Model file for the job. Use its own axes, mm. A direction names the side the tool comes from. Round coordinates to 2 decimals unless told otherwise and drop trailing zeros. Loops run counter-clockwise (first coordinate to the right, second up) from the corner with the lowest first, then second, coordinate; pieces in that order, holes last. Notation, with made-up numbers: (-0.75, 59) - (57.25, 59) arc R27 cw to (57.25, 86) - close; hole circle Ø1 at (21, 3). An arc over 180 degrees is marked (long way). Answer as a JSON object with one key per item and string values.
from build123d import *

# Parameters (mm, degrees)
F1_DEPTH = 127
F3_DEPTH = 177.8
F4_R     = 33.3375
F4_R_2   = 31.75
F5_DEPTH = 19.05
F6_T     = 7.62


# Not quite as in the source:
# - a shell that OpenCascade refuses in one call is made with other operations: the cavity is built on its own and cut out


with BuildPart() as f1:
    # F0 (on Right) → F1 (new body, symmetric)
    with BuildSketch(Plane.YZ):
        with BuildLine():
            Line((0, 76.4100525974), (0, 0))
            Line((0, 0), (671.8020987012, 0))
            ThreePointArc((671.8020987012, 0), (693.9200398628, 12.9117383606), (693.5512826501, 38.5199465532))
            Line((693.5512826501, 38.5199465532), (616.9399846733, 165.5199465532))
            ThreePointArc((616.9399846733, 165.5199465532), (607.6790623638, 174.5179411616), (595.1908007244, 177.8))
            Line((595.1908007244, 177.8), (434.3242754471, 177.8))
            add(Edge.make_bspline(
                [(434.3242754471, 177.8), (377.1008998353, 176.660223353), (237.5491375806, 169.4148859291), (92.7331109855, 131.2042560006), (30.2962614107, 107.6098996029), (13.6550616577, 98.9315184319)],
                knots=[0.1901896549, 0.1901896549, 0.1901896549, 0.1901896549, 0.3812653252, 0.674687688, 0.8202345165, 0.8202345165, 0.8202345165, 0.8202345165], degree=3))
            ThreePointArc((13.6550616577, 98.9315184319), (3.6804070723, 89.5789281398), (0, 76.4100525974))
        make_face()
    extrude(amount=F1_DEPTH, both=True)

    # F2 (on Top) → F3 (cut)
    with BuildSketch(Plane.XY):
        with BuildLine():
            Line((-127, 0), (-114.3, 0))
            Line((-114.3, 0), (-114.3, 220.98))
            ThreePointArc((-114.3, 220.98), (-118.0197438789, 229.9602561211), (-127, 233.68))
            Line((-127, 233.68), (-127, 0))
        make_face()
        with BuildLine():
            Line((114.3, 220.98), (114.3, 0))
            Line((114.3, 0), (127, 0))
            Line((127, 0), (127, 233.68))
            ThreePointArc((127, 233.68), (118.0197438789, 229.9602561211), (114.3, 220.98))
        make_face()
    extrude(amount=F3_DEPTH, mode=Mode.SUBTRACT)

    # F4 (on face) → F5 (join)
    with BuildSketch(Plane.XY.offset(177.8)):
        with Locations((60.96, 510.5242754471)):
            Circle(F4_R)
        with Locations((60.96, 510.5242754471)):
            Circle(F4_R_2, mode=Mode.SUBTRACT)
    extrude(amount=F5_DEPTH)

    # F6: shell of thickness 7.62, made by hand


with BuildPart() as f6_core1:
    # F6_t2: copy of F1
    add(f1.part)

    # the walls: a layer under each face that stays
    f6_faces = [f6_core1.faces().sort_by_distance(p)[0] for p in [
        (-63.5, 178.8934164203, 151.6082143397),
        (63.5, 178.8934164203, 151.6082143397),
        (0, 3.6804070723, 89.5789281398),
        (-114.3, 110.49, 79.9601525115),
        (-118.0197438789, 229.9602561211, 81.0374425071),
        (-127, 465.4410493506, 88.9),
        (0, 514.7575380857, 177.8),
        (114.3, 110.49, 79.9601525115),
        (118.0197438789, 229.9602561211, 81.0374425071),
        (127, 465.4410493506, 88.9),
        (0, 0, 38.2050262987),
        (0, 607.6790623638, 174.5179411616),
        (0, 655.2456336617, 102.0199465532),
        (0, 693.9200398628, 12.9117383606),
        (27.6225, 510.5242754471, 187.325),
        (29.845, 501.6342754471, 196.85),
        (29.21, 510.5242754471, 187.325),
        (60.96, 510.5242754471, 177.8),
    ]]
    thicken(f6_faces, amount=-F6_T, mode=Mode.SUBTRACT)

    # F6_s3 → F6_t4 (revolve, cut)
    with BuildSketch(Plane.XZ.offset(-510.5242754471)):
        Polygon((94.3737, 177.8762), (94.2975, 170.18), (86.6775, 170.18), (86.6775, 177.8), align=None)
    revolve(axis=Axis((60.96, 510.5242754471, 177.8), (0, 0, 1)), mode=Mode.SUBTRACT)

    # F6_s5 → F6_t6 (revolve, cut)
    with BuildSketch(Plane.XZ.offset(-510.5242754471)):
        Polygon((92.6338, 177.8762), (100.33, 177.8), (100.33, 170.18), (92.71, 170.18), align=None)
    revolve(axis=Axis((60.96, 510.5242754471, 177.8), (0, 0, 1)), mode=Mode.SUBTRACT)


with BuildPart() as f1_1:
    add(f1.part)

    # what is left inside the walls is the cavity
    f6_cavity = [f6_core1.part.solids().sort_by_distance(p)[0] for p in [
        (-39.793333, 339.711049, 0.0762),
    ]]
    add(f6_cavity, mode=Mode.SUBTRACT)


solid = f1_1.part
1) Drop flat-ended pins along their axis: P1, Ø5, axis at x = -55, z = 50.5, coming from the -Y side; P2, Ø12, axis at x = 96.5, y = 488.5, coming from the +Z side; P3, Ø4, axis at x = 43.5, y = 320, coming from the -Z side; P4, Ø3, axis at x = 38.5, z = 105.5, coming from the -Y side. Give the stop position or say it passes through.
Values follow:
{"P1": "y = 0", "P2": "z = 177.8", "P3": "z = 164.63", "P4": "y = 24.03"}
2) Two-plate mould, pull along X, no slides. Class faces 6 (the flat face through (123, 334, 0)), 7 (the flat face through (-114.3, 109, 61)), 8 (the cylindrical face through (1.494, 10.267, 85.744)): pulls with the +X half, pulls with the -X half, needs draft (parallel to the pull), parting line crosses it, or undercut.
Values follow:
{"face 6": "needs draft", "face 7": "pulls with the -X half", "face 8": "undercut"}
3) Probe probe 1 along Y at (x, z) = (60, 185); probe 2 along X at (y, z) = (181, 101); probe 3 along X at (y, z) = (507.5, 167). List the from-to ranges inside material, lowest first.
Values follow:
{"probe 1": "477.2 to 478.79, 542.26 to 543.85", "probe 2": "-114.3 to -106.68, 106.68 to 114.3", "probe 3": "-127 to -119.38, 119.38 to 127"}
4) Slice it at A-A on y = 653. List the corners of the cut face in (x, z), then the cut area to 3 significant figures.
Values follow:
{"outline": "(-127, 0) - (-119.38, 0) - (-119.38, 90.99) - (119.38, 90.99) - (119.38, 0) - (127, 0) - (127, 105.74) - (-127, 105.74) - close", "area": "5,130 mm²"}
5) Tool access for faces 1 (the flat face through (114.3, 112, 61)), 2 (the cylindrical face through (1.778, 607.838, 174.428)), 3 (the cylindrical face through (1.671, 687.154, 16.43)), 4 (the cylindrical face through (75.611, 482.357, 187.192)), 5 (the cylindrical face through (1.67, 604.04, 167.82)): list every direction of +Z, -Z, +X, -X, +Y, -Y with a clear straight run to the whole face (end or side of a thin tool).
Values follow:
{"face 1": "+Z, -Z, +X, -Y", "face 2": "+Z, +X, -X, +Y", "face 3": "none", "face 4": "+Z", "face 5": "-Z"}
